```python
from build123d import *

# Parameters (mm, degrees)
SKETCH1_W           = 85
SKETCH1_H           = 200
BOSS_EXTRUDE1_DEPTH = 5
FILLET1_R           = 1
SKETCH2_R           = 17.5
CUT_EXTRUDE1_DEPTH  = 2.5
FILLET2_R           = 0.125
SKETCH3_W           = 15
SKETCH3_H           = 85
BOSS_EXTRUDE2_DEPTH = 3
RIB1_START          = -5
RIB1_DEPTH          = 5
SKETCH5_R           = 1.5
CUT_EXTRUDE2_DEPTH  = 3
FILLET3_R           = 4
FILLET4_R           = 3


# Read off the part's stored shape, not the designer's step: Rib1
with BuildPart() as part:
    # Sketch1 → Boss-Extrude1 (new body)
    with BuildSketch(Plane(origin=(0, 0, 0), x_dir=(0, 0, -1), z_dir=(1, 0, 0))):
        with Locations((0, 100)):
            Rectangle(SKETCH1_W, SKETCH1_H)
        Polygon((-16, 25), (-16, 176), (-11, 176), (-11, 49), (-7, 49), (-7, 29), (-2.5, 29), (-2.5, 42), (16, 42), (16, 25), (16, 24), (15, 24), (-15, 24), (-16, 24), align=None, mode=Mode.SUBTRACT)
    extrude(amount=BOSS_EXTRUDE1_DEPTH)

    # Fillet1
    fillet1_edges = [part.edges().sort_by_distance(p)[0] for p in [
        (2.5, 42, 2.5),
        (2.5, 29, 2.5),
        (2.5, 29, 7),
        (2.5, 49, 11),
    ]]
    fillet(fillet1_edges, radius=FILLET1_R)

    # Sketch2 → Cut-Extrude1 (cut)
    with BuildSketch(Plane(origin=(5, 0, 0), x_dir=(0, 0, -1), z_dir=(1, 0, 0))):
        with Locations((15.75, 173.25)):
            Circle(SKETCH2_R)
        Polygon((15.75, 173.125), (15.625, 173.25), (8.75, 173.25), (15.75, 187.25), (15.75, 173.375), (15.875, 173.25), (22.75, 173.25), (15.75, 159.25), align=None, mode=Mode.SUBTRACT)
    extrude(amount=-CUT_EXTRUDE1_DEPTH, mode=Mode.SUBTRACT)

    # Fillet2
    fillet2_edges = [part.edges().sort_by_distance(p)[0] for p in [
        (3.75, 173.25, -15.625),
        (3.75, 173.125, -15.75),
        (3.75, 173.25, -15.875),
        (3.75, 173.375, -15.75),
    ]]
    fillet(fillet2_edges, radius=FILLET2_R)

    # Sketch3 → Boss-Extrude2 (add)
    with BuildSketch(Plane.XZ):
        with Locations((-7.5, 0)):
            Rectangle(SKETCH3_W, SKETCH3_H)
    extrude(amount=-BOSS_EXTRUDE2_DEPTH)

    # Rib1 outline → Rib1 (add)
    with BuildSketch(Plane.XY.offset(42.5).offset(RIB1_START)):
        Polygon((0, 18), (-15, 3), (0, 3), align=None)
    rib1 = extrude(amount=RIB1_DEPTH)

    # Mirror1: Rib1 across plane
    add(rib1.mirror(Plane.XY))

    # Sketch5 → Cut-Extrude2 (cut)
    with BuildSketch(Plane(origin=(0, 3, 0), x_dir=(1, 0, 0), z_dir=(0, 1, 0))):
        with Locations(Location((-7.5, 24.5, 0), (0, 0, 270))):
            Circle(SKETCH5_R)
        with Locations(Location((-7.5, 0, 0), (0, 0, 270))):
            Circle(SKETCH5_R)
        with Locations(Location((-7.5, -24.5, 0), (0, 0, 270))):
            Circle(SKETCH5_R)
    extrude(amount=-CUT_EXTRUDE2_DEPTH, mode=Mode.SUBTRACT)

    # Fillet3
    fillet3_edges = [part.edges().sort_by_distance(p)[0] for p in [
        (0, 18, 40),
        (0, 18, -40),
    ]]
    fillet(fillet3_edges, radius=FILLET3_R)

    # Fillet4
    fillet4_edges = [part.edges().sort_by_distance(p)[0] for p in [
        (0, 3, 0),
    ]]
    fillet(fillet4_edges, radius=FILLET4_R)


solid = part.part
```
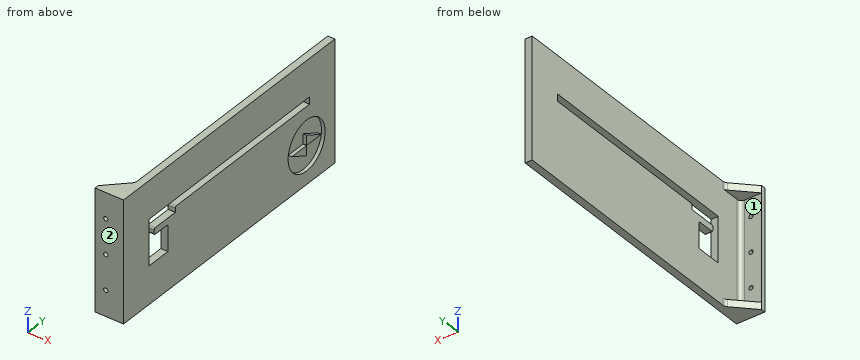
Model file for the job. Use its own axes, mm. Face numbers are marked on the shaded views. Coordinates: 2 decimals unless noted, no trailing zeros. Loops run counter-clockwise (first coordinate to the right, second up) from the corner with the lowest first, then second, coordinate; pieces in that order, holes last. Notation, with made-up numbers: (-36, -3) - (-27, -3) arc R28 cw to (-27, 23) - close; hole circle Ø3 at (63.5, 65). An arc over 180 degrees is marked (long way). Answer as a JSON object with one key per item and string values. Group by question number.
(1) Probe line 1 along Y through (x, z) = (1.75, -13); line 2 along X through (y, z) = (1.6, 0); line 3 along Z through (x, y) = (4.25, 183) (3 decimals). List the from-to ranges inside material, lowest first.
(2) Two-plate mould, pull along Z, no slides. Class the marked faces 1 and 2: released by +Z, released by -Z, zero draft, split by the parting line, or undercut.
(3) Flat gauge pins, fed straight in: pin 1 (6 mm diameter, centred on x = -9, z = 3.5, fed in from +Y); pin 2 (6 mm diameter, centred on x = -5, z = 6.5, fed in from +Y); pin 3 (6 mm diameter, centred on x = -4.5, z = 20.5, fed in from +Y). Where does each tip first touch, or does it go through?
(4) Cut at C-C (x = -13). Give the cut face in (y, z), then the cut area to 3 significant figures.
(5) Cut at B-B (y = 148). Give the cut face in (x, z), then the cut area to 3 significant figures.
(6) Cut at A-A (y = 32). Give the cut face in (x, z).
Geometry says:
{
 "1": {"line 1": "y = 0 to 24, 42 to 200", "line 2": "x = -15 to -9, -6 to 5", "line 3": "z = -42.5 to -30.282, -15.75 to -13.625, -1.218 to 42.5"},
 "2": {"face 1": "undercut", "face 2": "zero draft"},
 "3": {"pin 1": "stops at y = 3", "pin 2": "stops at y = 3.17", "pin 3": "stops at y = 3.4"},
 "4": {"outline": "(0, -42.5) - (5, -42.5) - (5, -37.5) - (3, -37.5) - (3, 37.5) - (5, 37.5) - (5, 42.5) - (0, 42.5) - close", "area": "275 mm^2"},
 "5": {"outline": "(0, -42.5) - (5, -42.5) - (5, 11) - (0, 11) - close; (0, 16) - (5, 16) - (5, 42.5) - (0, 42.5) - close", "area": "400 mm^2"},
 "6": {"outline": "(0, -42.5) - (5, -42.5) - (5, -16) - (0, -16) - close; (0, 2.5) - (5, 2.5) - (5, 7) - (0, 7) - close; (0, 16) - (5, 16) - (5, 42.5) - (0, 42.5) - close"}
}
